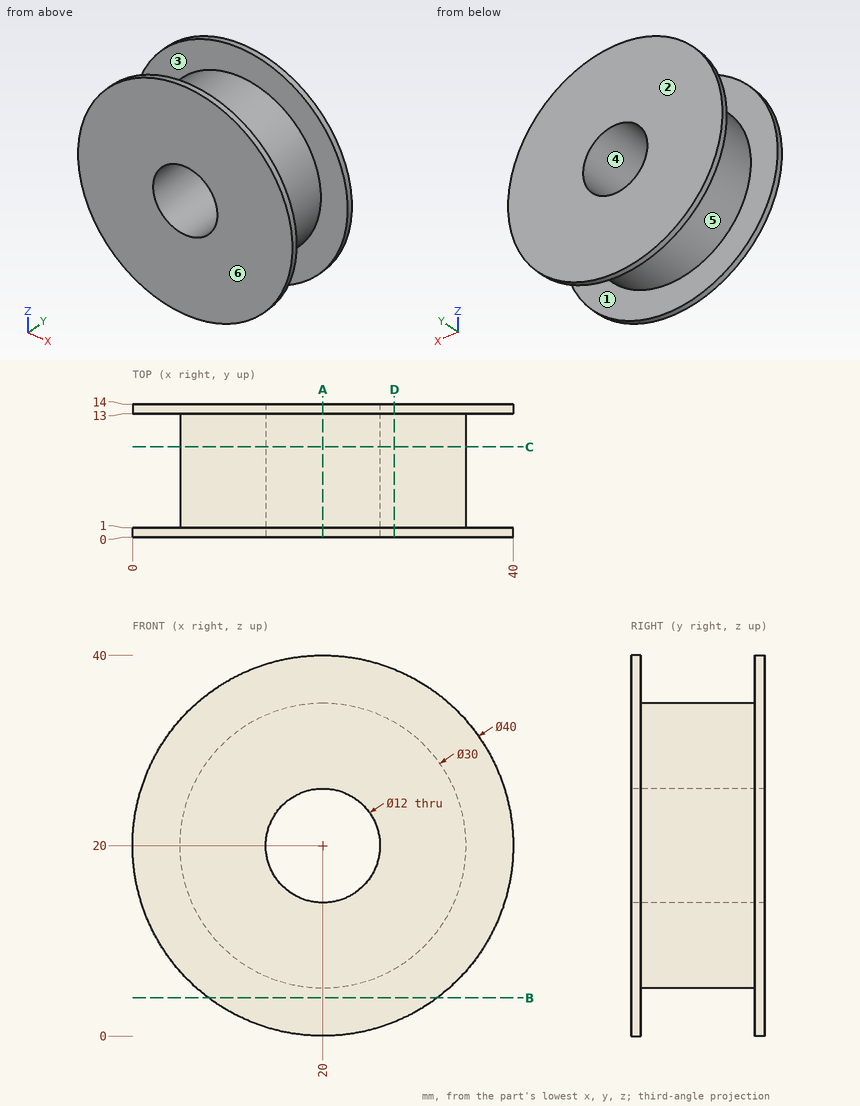
Design review of the part shown in the three views and the two pictorial views. Dimensions are in mm from the part's minimum x, y and z. A direction names the side the tool comes from. Round coordinates to 2 decimals unless told otherwise and drop trailing zeros. Write each loop counter-clockwise with the first axis right and the second up, starting at its lowest first coordinate (ties: lowest second). Pieces come first, ordered by that corner, then holes. Notation, with made-up numbers: M -27.75,29 L 18.25,29 A19 ccw 18.25,43 Z; hole C 73,26 d8. An arc over 180 degrees is marked long. Use a Markdown table: item, result. Add a question column.
Q1. We need section A-A, the plane x = 20. State the section outline as (y, z) points.
Q2. Machinability: for the marked faces 1 and 2, which of the approach directions +Z, -Z, +X, -X, +Y, -Y give a long, thin tool a straight path to every point of the face, cutting with its end or side? Answer none if there is none.
Q3. We need section B-B, the plane z = 4. State the section outline as (x, y) points, plus the area to 3 significant figures.
Q4. Insertion check: pin 1 (1 mm diameter, centred on y = 4, z = 10.5, fed in from +X); pin 2 (1.5 mm diameter, centred on x = 16, y = 2, fed in from -Z); pin 3 (1.5 mm diameter, centred on y = 7.5, z = 21.5, fed in from +X). Each pin has a flat end and moves straight along its axis. Give the tip position at first contact, or say it passes through.
Q5. We need section D-D, the plane x = 27.5. State the section outline as (y, z) points, plus the area to 3 significant figures.
Q6. The part is to be moulded in two halves that separate along Y. For the marked faces 3, 4, 5 and 6, say which applies: pulls with the +Y half, pulls with the -Y half, needs draft (parallel to the pull), parting line crosses it, or undercut.
Q7. To check wall thickness, follow line 1 (Y direction, x = 5, z = 12); line 2 (Z direction, x = 22.5, y = 5); line 3 (X direction, y = 5.75, z = 25). State the ranges of each line that lie inside material, in increasing order.
Q8. We need section C-C, the plane y = 9.5. State the section outline as (x, z) points, plus the area to 3 significant figures.
Findings below:
| question | item | result |
|---|---|---|
| 1 | outline | M 0,0 L 1,0 L 1,5 L 13,5 L 13,0 L 14,0 L 14,14 L 0,14 Z; M 0,26 L 14,26 L 14,40 L 13,40 L 13,35 L 1,35 L 1,40 L 0,40 Z |
| 2 | face 1 | none |
| 2 | face 2 | +Z, -Z, +X, -X, +Y |
| 3 | outline | M 8,0 L 32,0 L 32,1 L 8,1 Z; M 8,13 L 32,13 L 32,14 L 8,14 Z |
| 3 | area | 48.0 mm² |
| 4 | pin 1 | stops at x = 32 |
| 4 | pin 2 | stops at z = 5.36 |
| 4 | pin 3 | stops at x = 34.98 |
| 5 | outline | M 0,1.46 L 1,1.46 L 1,7.01 L 13,7.01 L 13,1.46 L 14,1.46 L 14,38.54 L 13,38.54 L 13,32.99 L 1,32.99 L 1,38.54 L 0,38.54 Z |
| 5 | area | 386 mm² |
| 6 | face 3 | undercut |
| 6 | face 4 | needs draft |
| 6 | face 5 | undercut |
| 6 | face 6 | pulls with the -Y half |
| 7 | line 1 | y = 0 to 1, 13 to 14 |
| 7 | line 2 | z = 5.21 to 14.55, 25.45 to 34.79 |
| 7 | line 3 | x = 5.86 to 16.68, 23.32 to 34.14 |
| 8 | outline | C 20,20 d30; hole C 20,20 d12 |
| 8 | area | 594 mm² |
